CAD build for the part. Positions are in the model's coordinates, mm. A direction names the side the tool comes from. Coordinates: 2 decimals unless noted, no trailing zeros. Write each loop counter-clockwise with the first axis right and the second up, starting at its lowest first coordinate (ties: lowest second). Pieces come first, ordered by that corner, then holes. Notation, with made-up numbers: (-30.5, 41) - (11.5, 41) arc R20 ccw to (11.5, 63) - close; hole circle Ø9 at (63.25, 4.5). An arc over 180 degrees is marked (long way). Answer in a Markdown table with one row per item. Add a question column.
Q1. 3-axis set-ups, long thin cutter, end or side, ignore diameter. For faces 1 (the flat face through (3.26, 4.77, 2.46)), 2 (the flat face through (1.74, 2.73, 2.46)), 3 (the flat face through (0.99, 2.19, 2.46)), 4 (the flat face through (3.986, 4.683, 2.465)): which of +Z, -Z, +X, -X, +Y, -Y reach the whole face in a straight line?
Q2. Drill centre lines: line 1 along Y through (x, z) = (2.95, 0.35); line 2 along Y through (x, z) = (4.5, 1.8); line 3 along Y through (x, z) = (2.35, 4.55). Where is each one in solid material? Low to high. Write a range as from..to.
Q3. Band-saw the part on A-A (y = 2.75). List the corners of the cut face in (x, z), and give its area (4 significant figures).
Q4. Two-plate mould, pull along X, no slides. Class faces 5 (the flat face through (1.74, 3.98, 2.46)), 6 (the flat face through (3.986, 3.433, 2.465)), 7 (the flat face through (1.74, 0.23, 2.46)), 8 (the flat face through (1.014, 0.317, 2.465)): +X half, -X half, draft (parallel to the pull), parting line (faces both ways), or undercut.
Q5. Band-saw the part on C-C (z = 0.7). State how many separate pieces and enclosed holes the cut face has, and give its area (4 significant figures).
Q6. Band-saw the part on D-D (x = 2.25). List the corners of the cut face in (y, z), and give its area (4 significant figures).
Q7. Band-saw the part on B-B (x = 4.1). List the corners of the cut face in (y, z).
```python
from build123d import *

# Parameters (mm, degrees)
BOSS_EXTRUDE2_DEPTH = 5


with BuildPart() as part:
    # Sketch1 → Boss-Extrude2 (new body)
    with BuildSketch(Plane.XY):
        Polygon((3, 0.625), (2.5, 0.46875), (4, 0), (5, 0), align=None)
        Polygon((4, 1.25), (2.5, 0.78125), (3, 0.625), (5, 1.25), (3, 1.875), (2.5, 1.71875), align=None)
        Polygon((2.5, 0.78125), (2, 0.625), (2.5, 0.46875), (3, 0.625), align=None)
        Polygon((2, 0.625), (0, 0), (1, 0), (2.5, 0.46875), align=None)
        Polygon((0, 1.25), (2, 0.625), (2.5, 0.78125), (1, 1.25), (2.5, 1.71875), (2, 1.875), align=None)
        Polygon((2.5, 2.03125), (2, 1.875), (2.5, 1.71875), (3, 1.875), align=None)
        Polygon((4, 2.5), (2.5, 2.03125), (3, 1.875), (5, 2.5), align=None)
        Polygon((0, 2.5), (2, 1.875), (2.5, 2.03125), (1, 2.5), align=None)
        Polygon((2.5, 2.96875), (4, 2.5), (5, 2.5), (3, 3.125), align=None)
        Polygon((2, 3.125), (0, 2.5), (1, 2.5), (2.5, 2.96875), align=None)
        Polygon((2.5, 3.28125), (2, 3.125), (2.5, 2.96875), (3, 3.125), align=None)
        Polygon((0, 3.75), (2, 3.125), (2.5, 3.28125), (1, 3.75), (2.5, 4.21875), (2, 4.375), align=None)
        Polygon((4, 3.75), (2.5, 3.28125), (3, 3.125), (5, 3.75), (3, 4.375), (2.5, 4.21875), align=None)
        Polygon((2.5, 4.53125), (2, 4.375), (2.5, 4.21875), (3, 4.375), align=None)
        Polygon((0, 5), (2, 4.375), (2.5, 4.53125), (1, 5), align=None)
        Polygon((4, 5), (2.5, 4.53125), (3, 4.375), (5, 5), align=None)
    extrude(amount=BOSS_EXTRUDE2_DEPTH)


solid = part.part
```
Checked values:
| question | item | result |
|---|---|---|
| 1 | face 1 | +Z, -Z, +Y |
| 1 | face 2 | +Z, -Z |
| 1 | face 3 | +Z, -Z, -X |
| 1 | face 4 | +Z, -Z, +X |
| 2 | line 1 | y = 0.33..0.92, 1.58..2.17, 2.83..3.42, 4.08..4.67 |
| 2 | line 2 | y = 0..0.16, 1.09..1.41, 2.34..2.66, 3.59..3.91, 4.84..5 |
| 2 | line 3 | y = 0.42..0.83, 1.67..2.08, 2.92..3.33, 4.17..4.58 |
| 3 | outline | (0.8, 0) - (1.8, 0) - (1.8, 5) - (0.8, 5) - close; (3.2, 0) - (4.2, 0) - (4.2, 5) - (3.2, 5) - close |
| 3 | area | 10.00 mm² |
| 4 | face 5 | undercut |
| 4 | face 6 | +X half |
| 4 | face 7 | undercut |
| 4 | face 8 | -X half |
| 5 | separate pieces | 1 |
| 5 | enclosed holes | 3 |
| 5 | area | 9.375 mm² |
| 6 | outline | (0.39, 0) - (0.86, 0) - (0.86, 5) - (0.39, 5) - close; (1.64, 0) - (2.11, 0) - (2.11, 5) - (1.64, 5) - close; (2.89, 0) - (3.36, 0) - (3.36, 5) - (2.89, 5) - close; (4.14, 0) - (4.61, 0) - (4.61, 5) - (4.14, 5) - close |
| 6 | area | 9.375 mm² |
| 7 | outline | (0, 0) - (0.28, 0) - (0.28, 5) - (0, 5) - close; (0.97, 0) - (1.53, 0) - (1.53, 5) - (0.97, 5) - close; (2.22, 0) - (2.78, 0) - (2.78, 5) - (2.22, 5) - close; (3.47, 0) - (4.03, 0) - (4.03, 5) - (3.47, 5) - close; (4.72, 0) - (5, 0) - (5, 5) - (4.72, 5) - close |
